The model under review builds one solid part; all positions refer to its coordinate system, in mm. A direction names the side the tool comes from. Give positions to 0.01 mm unless a question says otherwise; leave off trailing zeros. Write each loop counter-clockwise with the first axis right and the second up, starting at its lowest first coordinate (ties: lowest second). Pieces come first, ordered by that corner, then holes.
from build123d import *

# Parameters (mm, degrees)
F0_W          = 71.3502541184
F0_H          = 47.3797805607
F1_DEPTH      = 25.4
F1_TAPER      = -3
F1_DEPTH_BACK = 25.4


with BuildPart() as f1:
    # F0 (on Top) → F1 (new body, two sides)
    with BuildSketch(Plane.XY) as f1_sk:
        with Locations((35.6751270592, 23.6898902804)):
            Rectangle(F0_W, F0_H)
    extrude(amount=F1_DEPTH, taper=F1_TAPER)
    extrude(f1_sk.sketch, amount=-F1_DEPTH_BACK)


solid = f1.part
1) Consider section A-A, the plane z = -17. Give the boundary of the cut face in (x, y).
2) Tool access review of faces 1 (the flat face through (0, 23, -13)), 2 (the flat face through (71.35, 23, -13)), 3 (the flat face through (35, 47.38, -13)), 4 (the flat face through (35, 0, -13)): name each direction out of +Z, -Z, +X, -X, +Y, -Y from which nothing blocks a thin tool from reaching the whole face with its end or side.
3) Insertion check: pin 1 (6 mm diameter, centred on y = 39, z = 5.5, fed in from -X); pin 2 (20.5 mm diameter, centred on x = 33.5, z = -16.5, fed in from -Y); pin 3 (1.5 mm diameter, centred on x = 24, z = -18, fed in from +Y). Each pin has a flat end and moves straight along its axis. Give the tip position at first contact, or say it passes through.
4) To check wall thickness, follow probe 1 along X at (y, z) = (31, -20); probe 2 along Y at (x, z) = (12.5, -11.5); probe 3 along X at (y, z) = (41, 3). State the ranges of each line that lie inside material, in increasing order.
Answer block:
1. outline: (0, 0) - (71.35, 0) - (71.35, 47.38) - (0, 47.38) - close
2. face 1: -Z, -X, +Y, -Y
2. face 2: -Z, +X, +Y, -Y
2. face 3: -Z, +X, -X, +Y
2. face 4: -Z, +X, -X, -Y
3. pin 1: stops at x = -0.45
3. pin 2: stops at y = 0
3. pin 3: stops at y = 47.38
4. probe 1: x = 0 to 71.35
4. probe 2: y = 0 to 47.38
4. probe 3: x = -0.16 to 71.51
